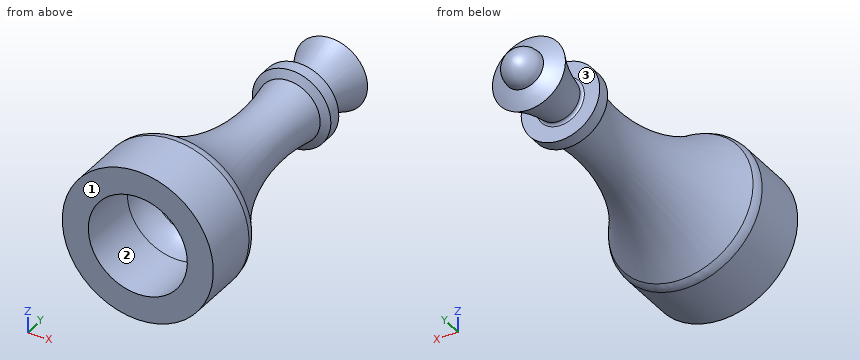
```python
from build123d import *

# Parameters (mm, degrees)
FILLET1_R = 3
FILLET2_R = 0.5


with BuildPart() as part:
    # Sketch1 → Revolve2 (revolve)
    with BuildSketch(Plane.XY, mode=Mode.PRIVATE) as revolve2_sk:
        with BuildLine():
            Line((9.5, 12), (9.5, 0))
            Line((9.5, 0), (14.5, 0))
            Line((14.5, 0), (14.5, 12))
            ThreePointArc((14.5, 12), (6.46129463, 28.348941445), (6, 46.56146125))
            Line((6, 46.56146125), (7.536573788, 47.396000215))
            Line((7.536573788, 47.396000215), (7.536573788, 49.844035403))
            Line((7.536573788, 49.844035403), (4.016092882, 49.844035403))
            ThreePointArc((4.016092882, 49.844035403), (5.09741657, 54.8289558), (7.005928337, 59.559312565))
            ThreePointArc((7.005928337, 59.559312565), (5.43849666, 60.452627999), (3.765468303, 61.127780309))
            ThreePointArc((3.765468303, 61.127780309), (2.684487968, 63.843540801), (0, 65))
            Line((0, 65), (0, 30))
            Line((0, 30), (8.006428895, 17.203147345))
            ThreePointArc((8.006428895, 17.203147345), (9.11921693, 14.706635224), (9.5, 12))
        make_face()
    revolve(revolve2_sk.sketch.rotate(Axis((0, 0, 0), (0, 1, 0)), 90), axis=Axis((0, 0, 0), (0, 1, 0)))

    # Fillet1
    fillet1_edges = [part.edges().sort_by_distance(p)[0] for p in [
        (0, 12, 14.5),
    ]]
    fillet(fillet1_edges, radius=FILLET1_R)

    # Fillet2
    fillet2_edges = [part.edges().sort_by_distance(p)[0] for p in [
        (0, 49.844035403, 4.016092882),
    ]]
    fillet(fillet2_edges, radius=FILLET2_R)


solid = part.part
```
CAD build for the part. Positions are in the model's coordinates, mm. Face numbers are marked on the shaded views. Coordinates: 2 decimals unless noted, no trailing zeros. Order: outer loops, then holes, each group sorted by start corner. A loop starts at its lowest first (then second) coordinate and runs counter-clockwise, first axis right, second up. Notation, with made-up numbers: (-14, 9) - (8, 9) arc R23 cw to (8, 47) - close; hole circle Ø4 at (0.5, 44.5). An arc over 180 degrees is marked (long way). Use a Markdown table: item, result. Add a question column.
(1) Pull direction Y, two halves, no side cores. Call the marked faces 1, 2 and 3: +Y half, -Y half, draft (parallel to the pull), parting line (faces both ways), or undercut.
(2) Saw through at D-D (y = 55). Give the cut face in (x, z), then the cut area to 3 significant figures.
(3) Saw through at B-B (y = 38.5). Give the cut face in (x, z), then the cut area to 3 significant figures.
(4) Drill centre lines: line 1 along X through (y, z) = (7.25, 0); line 2 along Z through (x, y) = (-3.75, 41); line 3 along Z through (x, y) = (1.5, 24). Where is each one in solid material? Low to high. Write a range as [from, to].
(5) Flat gauge pins, fed straight in: pin 1 (6 mm diameter, centred on x = -4.5, y = 14.5, fed in from -Z); pin 2 (4 mm diameter, centred on x = -3.5, y = 53.5, fed in from +Z); pin 3 (2 mm diameter, centred on x = -4, z = 4.5, fed in from -Y). Where does each tip first touch, or does it go through?
(6) Saw through at A-A (y = 24). Give the cut face in (x, z), then the cut area to 3 significant figures.
(7) Saw through at C-C (y = 4). Give the cut face in (x, z), then the cut area to 3 significant figures.
Solved:
| question | item | result |
|---|---|---|
| 1 | face 1 | -Y half |
| 1 | face 2 | draft |
| 1 | face 3 | undercut |
| 2 | outline | circle Ø10.3 at (0, 0) |
| 2 | area | 83.3 mm² |
| 3 | outline | circle Ø10.46 at (0, 0) |
| 3 | area | 85.9 mm² |
| 4 | line 1 | x = [-14.5, -9.5], [9.5, 14.5] |
| 4 | line 2 | z = [-3.75, 3.75] |
| 4 | line 3 | z = [-7.63, -3.44], [3.44, 7.63] |
| 5 | pin 1 | stops at z = -14.04 |
| 5 | pin 2 | stops at z = 4.69 |
| 5 | pin 3 | stops at y = 18.78 |
| 6 | outline | circle Ø15.56 at (0, 0); hole circle Ø7.51 at (0, 0) |
| 6 | area | 146 mm² |
| 7 | outline | circle Ø29 at (0, 0); hole circle Ø19 at (0, 0) |
| 7 | area | 377 mm² |
